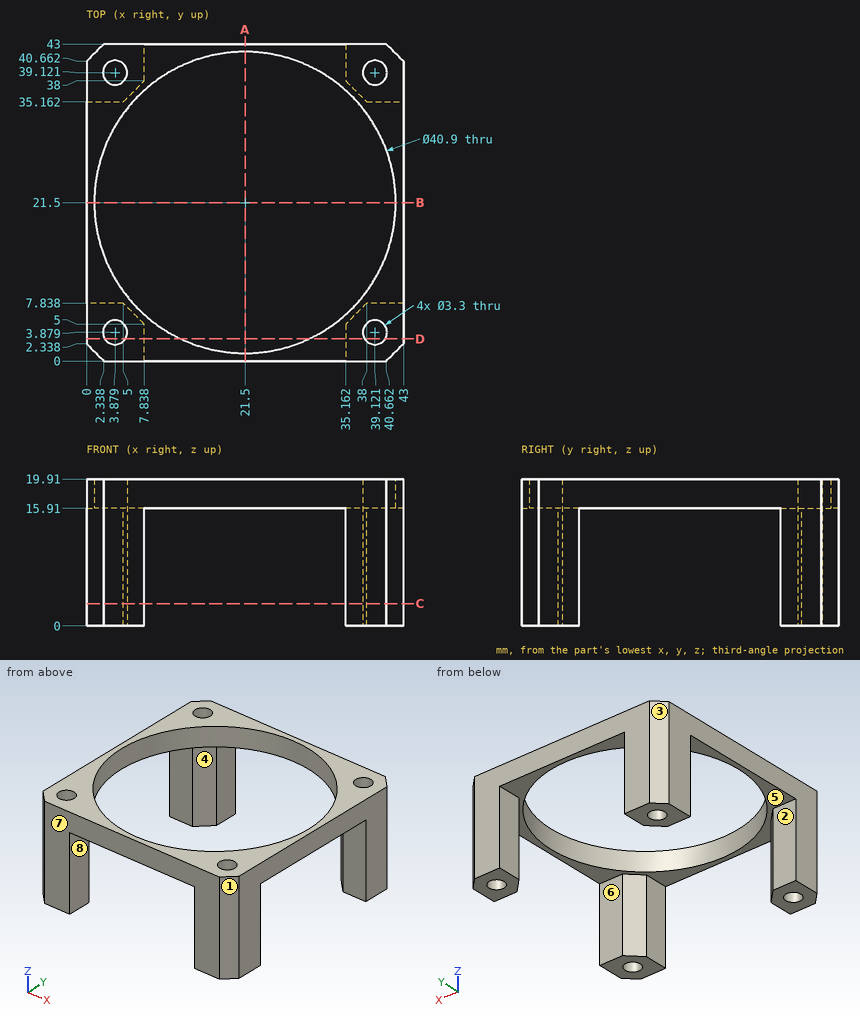
Geometry check sheet. Reference: drawing and pictorial views, mm from the part's lowest x, y, z. A direction names the side the tool comes from. Give positions to 0.01 mm unless a question says otherwise; leave off trailing zeros. Order: outer loops, then holes, each group sorted by start corner. A loop starts at its lowest first (then second) coordinate and runs counter-clockwise, first axis right, second up. Notation, with made-up numbers: M -7,24 L 36,24 A21 cw 36,51 Z; hole C 54.25,27.25 d2. An arc over 180 degrees is marked long. Answer in a Markdown table with one row per item. Add a question column.
Item 1: Tool access check on the marked faces 5, 6, 7 and 8. Record the directions out of +Z, -Z, +X, -X, +Y, -Y that give a thin tool (end or side, any length) a straight path to the whole face; none if there is none.
Item 2: Scan lines: probe 1 along Y at (x, z) = (4, 7.75); probe 2 along Y at (x, z) = (40.5, 14.5) (1 decimal); probe 3 along X at (y, z) = (38.5, 1.25). Record each from-to range of solid material in increasing order. Write a range as from..to.
Item 3: Section check D-D, the plane y = 3. Enter the section's corners in (x, z) (1 decimal).
Item 4: Section check C-C, the plane z = 3. Enter the section's corners in (x, y).
Item 5: Section check A-A, the plane x = 21.5. Enter the section's corners in (y, z).
Item 6: Mould release check, pull along X, two halves, no side actions. Record for the marked faces 1, 2, 3 and 4: released by +X, released by -X, zero draft, split by the parting line, or undercut.
Filled sheet:
| question | item | result |
|---|---|---|
| 1 | face 5 | -Z |
| 1 | face 6 | -Z, +X, -X |
| 1 | face 7 | +Z, -Z, +X, -X, -Y |
| 1 | face 8 | -Z, +Y, -Y |
| 2 | probe 1 | y = 0..2.23, 5.52..7.84, 35.16..37.48, 40.77..43 |
| 2 | probe 2 | y = 0..3, 4.8..7.8, 35.2..38.2, 40..43 |
| 2 | probe 3 | x = 0..2.35, 5.41..7.84, 35.16..37.59, 40.65..43 |
| 3 | outline | M 0,0 L 2.5,0 L 2.5,19.9 L 0,19.9 Z; M 5.3,0 L 7.8,0 L 7.8,15.9 L 12.8,15.9 L 12.8,19.9 L 5.3,19.9 Z; M 30.2,15.9 L 35.2,15.9 L 35.2,0 L 37.7,0 L 37.7,19.9 L 30.2,19.9 Z; M 40.5,0 L 43,0 L 43,19.9 L 40.5,19.9 Z |
| 4 | outline | M 0,2.34 L 2.34,0 L 7.84,0 L 7.84,5 L 5,7.84 L 0,7.84 Z; M 0,35.16 L 5,35.16 L 7.84,38 L 7.84,43 L 2.34,43 L 0,40.66 Z; M 35.16,0 L 40.66,0 L 43,2.34 L 43,7.84 L 38,7.84 L 35.16,5 Z; M 35.16,38 L 38,35.16 L 43,35.16 L 43,40.66 L 40.66,43 L 35.16,43 Z; hole C 3.88,3.88 d3.3; hole C 3.88,39.12 d3.3; hole C 39.12,3.88 d3.3; hole C 39.12,39.12 d3.3 |
| 5 | outline | M 0,15.91 L 1.05,15.91 L 1.05,19.91 L 0,19.91 Z; M 41.95,15.91 L 43,15.91 L 43,19.91 L 41.95,19.91 Z |
| 6 | face 1 | released by +X |
| 6 | face 2 | zero draft |
| 6 | face 3 | released by -X |
| 6 | face 4 | undercut |
